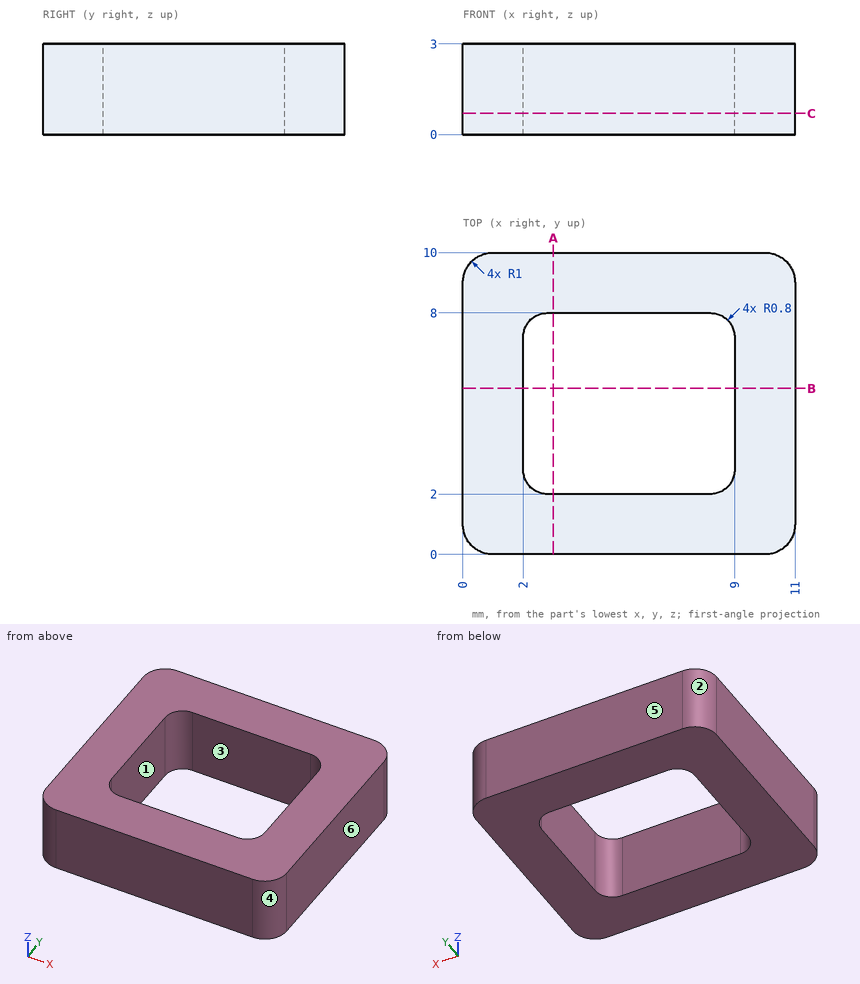
Check sheet for the drawn part. Datum: minimum x, y, z corner. Units: mm. A direction names the side the tool comes from. Give positions to 0.01 mm unless a question says otherwise; leave off trailing zeros. Loops run counter-clockwise (first coordinate to the right, second up) from the corner with the lowest first, then second, coordinate; pieces in that order, holes last.
1) Sectioned sample at B-B, the plane y = 5.5. Enter the section's corners in (x, z).
2) Depth check by flat-ended pin: pin 1 Ø5 at (x, y) = (7, 5) entering from -Z. Enter the tip coordinate at first touch or a pass-through.
3) Set-up check for the marked faces 1 and 2: record each of +Z, -Z, +X, -X, +Y, -Y from which the full face is reachable in a straight line by a thin tool's end or side.
4) Sectioned sample at A-A, the plane x = 3. Enter the section's corners in (y, z).
5) Thickness scan on line 1 along Y through (x, z) = (8.25, 2.4); line 2 along X through (y, z) = (6.75, 1.5); line 3 along Y through (x, z) = (10.5, 0.35). Record the ranges inside material, lowest first.
6) Sectioned sample at C-C, the plane z = 0.7. Enter the section's corners in (x, y).
7) Draft check along Y on the marked faces 3, 4, 5 and 6. Enter one of: pulls with the +Y half, pulls with the -Y half, needs draft (parallel to the pull), parting line crosses it, or undercut.
Answers:
1. outline: (0, 0) - (2, 0) - (2, 3) - (0, 3) - close; (9, 0) - (11, 0) - (11, 3) - (9, 3) - close
2. pin 1: stops at z = 0
3. face 1: +Z, -Z
3. face 2: +Z, -Z, -X, +Y
4. outline: (0, 0) - (2, 0) - (2, 3) - (0, 3) - close; (8, 0) - (10, 0) - (10, 3) - (8, 3) - close
5. line 1: y = 0 to 2, 8 to 10
5. line 2: x = 0 to 2, 9 to 11
5. line 3: y = 0.13 to 9.87
6. outline: (0, 1) arc R1 ccw to (1, 0) - (10, 0) arc R1 ccw to (11, 1) - (11, 9) arc R1 ccw to (10, 10) - (1, 10) arc R1 ccw to (0, 9) - close; hole (2, 2.8) arc R0.8 ccw to (2.8, 2) - (8.2, 2) arc R0.8 ccw to (9, 2.8) - (9, 7.2) arc R0.8 ccw to (8.2, 8) - (2.8, 8) arc R0.8 ccw to (2, 7.2) - close
7. face 3: undercut
7. face 4: pulls with the -Y half
7. face 5: pulls with the +Y half
7. face 6: needs draft
